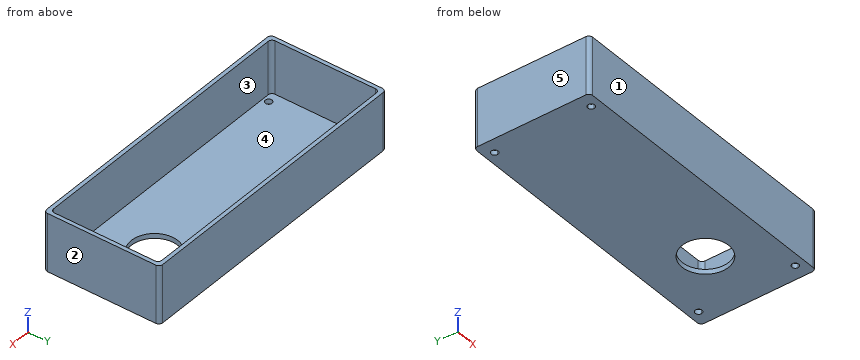
```python
from build123d import *

# Parameters (mm, degrees)
F0_W     = 150
F0_H     = 60
F1_DEPTH = 2.5
F2_W     = 150
F2_H     = 60
F2_W_2   = 146
F2_H_2   = 56
F3_DEPTH = 30
F4_R     = 2


with BuildPart() as f1:
    # F0 (on Top) → F1 (new body)
    with BuildSketch(Plane.XY):
        Rectangle(F0_W, F0_H)
        with BuildLine():
            ThreePointArc((-65.75, -25), (-68.7374368671, -26.2374368671), (-67.5, -23.25))
            ThreePointArc((-67.5, -23.25), (-66.2625631329, -23.7625631329), (-65.75, -25))
        make_face(mode=Mode.SUBTRACT)
        with BuildLine():
            ThreePointArc((69.25, -25), (66.2625631329, -26.2374368671), (67.5, -23.25))
            ThreePointArc((67.5, -23.25), (68.7374368671, -23.7625631329), (69.25, -25))
        make_face(mode=Mode.SUBTRACT)
        with BuildLine():
            ThreePointArc((-65.75, 25), (-66.2625631329, 23.7625631329), (-67.5, 23.25))
            ThreePointArc((-67.5, 23.25), (-68.7374368671, 26.2374368671), (-65.75, 25))
        make_face(mode=Mode.SUBTRACT)
        with BuildLine():
            ThreePointArc((52, 0), (40, -12), (28, 0))
            ThreePointArc((28, 0), (40, 12), (52, 0))
        make_face(mode=Mode.SUBTRACT)
        with BuildLine():
            ThreePointArc((69.25, 25), (68.7374368671, 23.7625631329), (67.5, 23.25))
            ThreePointArc((67.5, 23.25), (66.2625631329, 26.2374368671), (69.25, 25))
        make_face(mode=Mode.SUBTRACT)
    extrude(amount=F1_DEPTH)

    # F2 (on Top) → F3 (join)
    with BuildSketch(Plane.XY):
        Rectangle(F2_W, F2_H)
        Rectangle(F2_W_2, F2_H_2, mode=Mode.SUBTRACT)
    extrude(amount=F3_DEPTH)

    # F4
    f4_edges = [f1.edges().sort_by_distance(p)[0] for p in [
        (-73, 28, 16.25),
        (73, 28, 16.25),
        (-73, -28, 16.25),
        (73, -28, 16.25),
        (-75, 30, 15),
        (-75, -30, 15),
        (75, -30, 15),
        (75, 30, 15),
    ]]
    fillet(f4_edges, radius=F4_R)


solid = f1.part
```
Model file for the job. Use its own axes, mm. Face numbers are marked on the shaded views. A direction names the side the tool comes from. Round coordinates to 2 decimals unless told otherwise and drop trailing zeros. Write each loop counter-clockwise with the first axis right and the second up, starting at its lowest first coordinate (ties: lowest second). Pieces come first, ordered by that corner, then holes. Notation, with made-up numbers: (-14.5, 20.5) - (18.5, 20.5) arc R20 cw to (18.5, 39.5) - close; hole circle Ø2 at (14.25, 28). An arc over 180 degrees is marked (long way). Use CSV: the item, a comma, the result in double quotes. Start each with the question number.
Item 1: Band-saw the part on C-C (x = -27). Write the cut outline in (y, z).
Item 2: Two-plate mould, pull along X, no slides. Class the marked faces 1, 2 and 3: released by +X, released by -X, zero draft, split by the parting line, or undercut.
Item 3: Pin check, flat tips, straight feed: P1, Ø4, axis at x = 67.5, y = -25, coming from the +Z side; P2, Ø3, axis at x = -67.5, y = -25, coming from the +Z side. Stop position of each tip, or through.
Item 4: Drill centre lines: L1, parallel to X at y = 25, z = 0.75; L2, parallel to Y at x = -67.5, z = 2; L3, parallel to Y at x = -56.5, z = 23.75. Where is each one in solid material? Low to high. Write a range as [from, to].
Item 5: Tool access for the marked faces 4 and 5: list every direction of +Z, -Z, +X, -X, +Y, -Y with a clear straight run to the whole face (end or side of a thin tool).
Item 6: Band-saw the part on A-A (y = 0). Write the cut outline in (x, z), and give its area (3 significant figures).
Item 7: Band-saw the part on D-D (y = -17.5). Write the cut outline in (x, z).
Item 8: Band-saw the part on B-B (z = 23.5). Write the cut outline in (x, y), and give its area (3 significant figures).
Checked values:
1,outline,"(-30, 0) - (30, 0) - (30, 30) - (28, 30) - (28, 2.5) - (-28, 2.5) - (-28, 30) - (-30, 30) - close"
2,face 1,"zero draft"
2,face 2,"released by +X"
2,face 3,"undercut"
3,P1,"stops at z = 2.5"
3,P2,"passes through"
4,L1,"x = [-75, -69.25], [-65.75, 65.75], [69.25, 75]"
4,L2,"y = [-30, -26.75], [-23.25, 23.25], [26.75, 30]"
4,L3,"y = [-30, -28], [28, 30]"
5,face 4,"+Z"
5,face 5,"+Z, -Z, -X, +Y, -Y"
6,outline,"(-75, 0) - (28, 0) - (28, 2.5) - (-73, 2.5) - (-73, 30) - (-75, 30) - close; (52, 0) - (75, 0) - (75, 30) - (73, 30) - (73, 2.5) - (52, 2.5) - close"
6,area,"425 mm²"
7,outline,"(-75, 0) - (75, 0) - (75, 30) - (73, 30) - (73, 2.5) - (-73, 2.5) - (-73, 30) - (-75, 30) - close"
8,outline,"(-75, -28) arc R2 ccw to (-73, -30) - (73, -30) arc R2 ccw to (75, -28) - (75, 28) arc R2 ccw to (73, 30) - (-73, 30) arc R2 ccw to (-75, 28) - close; hole (-73, -26) arc R2 ccw to (-71, -28) - (71, -28) arc R2 ccw to (73, -26) - (73, 26) arc R2 ccw to (71, 28) - (-71, 28) arc R2 ccw to (-73, 26) - close"
8,area,"824 mm²"
